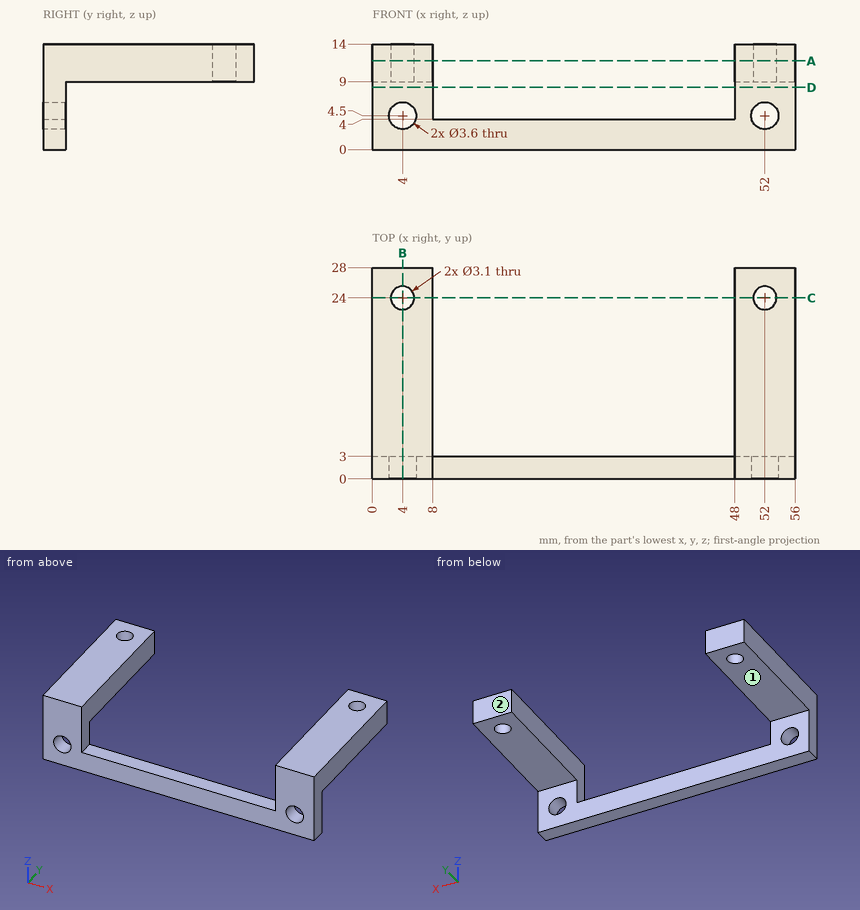
Verification items for this drawing (mm, ordinates from the low corner). A direction names the side the tool comes from. Coordinates: 2 decimals unless noted, no trailing zeros. Loops run counter-clockwise (first coordinate to the right, second up) from the corner with the lowest first, then second, coordinate; pieces in that order, holes last. Notation, with made-up numbers: (-10, -39) -> (16, -39) arc R27 cw to (16, -10) -> close; hole circle Ø11 at (-39, -23). An arc over 180 degrees is marked (long way). Answer in a Markdown table with one row per item. Add a question column.
1. Section check A-A, the plane z = 11.75. Enter the section's corners in (x, y).
2. Section check D-D, the plane z = 8.25. Enter the section's corners in (x, y).
3. Access from +Z, -Z, +X, -X, +Y, -Y to the whole of each face (thin tool, end or side, straight path). Record for the marked faces 1 and 2.
4. Material ranges on probe 1 along X at (y, z) = (7.5, 9.25); probe 2 along Y at (x, z) = (4, 13.75); probe 3 along X at (y, z) = (24.5, 12), recorded low to high. Write a range as [from, to].
5. Depth check by flat-ended pin: P1, Ø1.5, axis at x = 27.5, y = 2, coming from the +Z side; P2, Ø2.5, axis at x = 52, y = 24, coming from the -Z side; P3, Ø2.5, axis at x = 5.5, y = 19.5, coming from the -Z side; P4, Ø4, axis at x = 4, z = 4.5, coming from the +Y side. Enter the tip coordinate at first touch or a pass-through.
6. Section check B-B, the plane x = 4. Enter the section's corners in (y, z).
7. Section check C-C, the plane y = 24. Enter the section's corners in (x, z).
Derived:
| question | item | result |
|---|---|---|
| 1 | outline | (0, 0) -> (8, 0) -> (8, 28) -> (0, 28) -> close; (48, 0) -> (56, 0) -> (56, 28) -> (48, 28) -> close; hole circle Ø3.1 at (4, 24); hole circle Ø3.1 at (52, 24) |
| 2 | outline | (0, 0) -> (8, 0) -> (8, 3) -> (0, 3) -> close; (48, 0) -> (56, 0) -> (56, 3) -> (48, 3) -> close |
| 3 | face 1 | -Z, +X, -X, +Y |
| 3 | face 2 | +Z, -Z, +X, -X, +Y |
| 4 | probe 1 | x = [0, 8], [48, 56] |
| 4 | probe 2 | y = [0, 22.45], [25.55, 28] |
| 4 | probe 3 | x = [0, 2.53], [5.47, 8], [48, 50.53], [53.47, 56] |
| 5 | P1 | stops at z = 4 |
| 5 | P2 | passes through |
| 5 | P3 | stops at z = 9 |
| 5 | P4 | stops at y = 3 |
| 6 | outline | (0, 0) -> (3, 0) -> (3, 2.7) -> (0, 2.7) -> close; (0, 6.3) -> (3, 6.3) -> (3, 9) -> (22.45, 9) -> (22.45, 14) -> (0, 14) -> close; (25.55, 9) -> (28, 9) -> (28, 14) -> (25.55, 14) -> close |
| 7 | outline | (0, 9) -> (2.45, 9) -> (2.45, 14) -> (0, 14) -> close; (5.55, 9) -> (8, 9) -> (8, 14) -> (5.55, 14) -> close; (48, 9) -> (50.45, 9) -> (50.45, 14) -> (48, 14) -> close; (53.55, 9) -> (56, 9) -> (56, 14) -> (53.55, 14) -> close |
